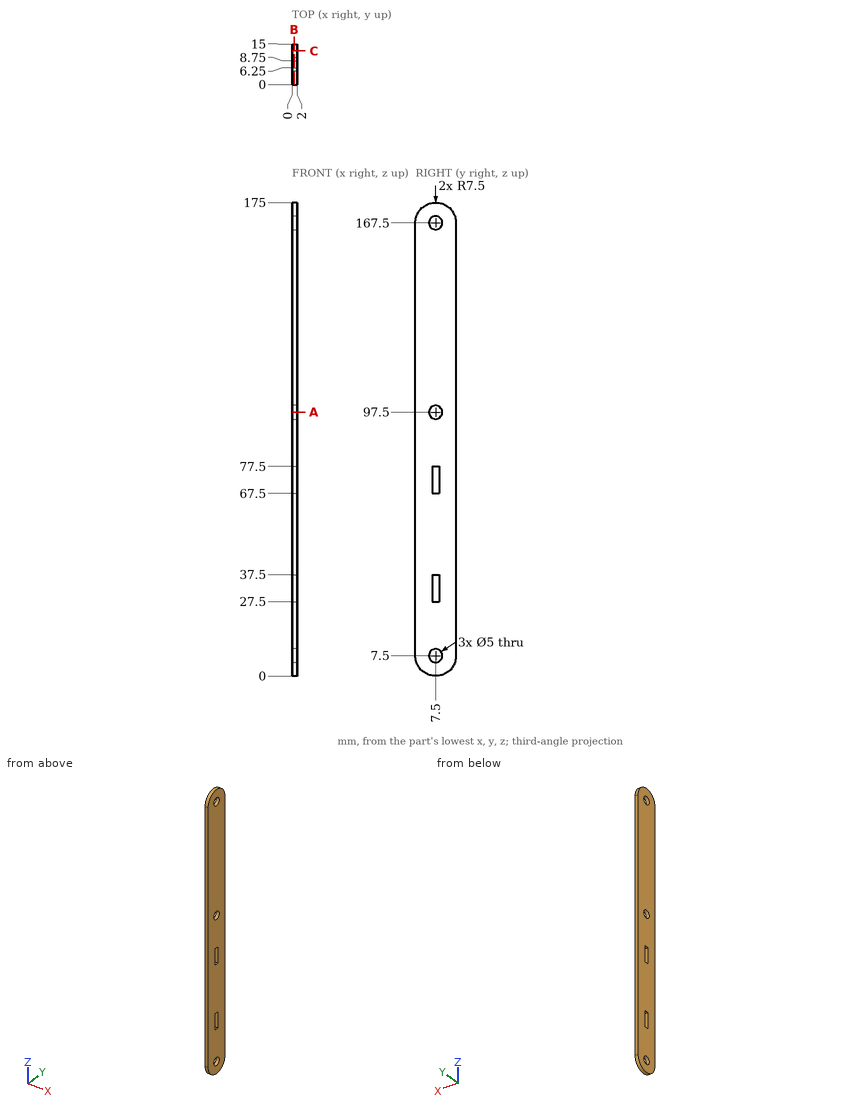
Source: three-view drawing plus pictorial views. Frame: mm from the lowest corner of the part. Give positions to 0.01 mm unless a question says otherwise; leave off trailing zeros. Write each loop counter-clockwise with the first axis right and the second up, starting at its lowest first coordinate (ties: lowest second). Pieces come first, ordered by that corner, then holes. Notation, with made-up numbers: (-10.5, 70) - (32.5, 70) arc R25 ccw to (32.5, 92) - close; hole circle Ø2 at (-34, 64). An arc over 180 degrees is marked (long way). Write item = value, one per line. Start each with the question number.
Q1. Cut plane B-B, the plane x = 0.75. Return loops of the section in (y, z), then the cut area to 3 significant figures.
Q2. Material intervals for probe 1 along Y at (x, z) = (1.1, 167.5); probe 2 along Z at (x, y) = (0.75, 6); probe 3 along Y at (x, z) = (0.15, 28), sorted ascending.
Q3. Cut plane C-C, the plane y = 12.5. Return loops of the section in (x, z), then the cut area to 3 significant figures.
Q4. Pin query (flat end, axial travel): pin 1 Ø0.6 at (x, y) = (1, 8) entering from -Z; pin 2 Ø6.5 at (y, z) = (7.5, 97.5) entering from +X. Return the tip coordinate at first contact, or that it passes through.
Q5. Cut plane A-A, the plane z = 97.5. Return loops of the section in (x, y).
Computed values:
q1.outline = (0, 7.5) arc R7.5 ccw to (15, 7.5) - (15, 167.5) arc R7.5 ccw to (0, 167.5) - close; hole circle Ø5 at (7.5, 7.5); hole circle Ø5 at (7.5, 97.5); hole circle Ø5 at (7.5, 167.5); hole (6.25, 27.5) - (8.75, 27.5) - (8.75, 37.5) - (6.25, 37.5) - close; hole (6.25, 67.5) - (8.75, 67.5) - (8.75, 77.5) - (6.25, 77.5) - close
q1.area = 2,470 mm²
q2.probe_1 = 0 to 5, 10 to 15
q2.probe_2 = 0.15 to 5.5, 9.5 to 95.5, 99.5 to 165.5, 169.5 to 174.85
q2.probe_3 = 0 to 6.25, 8.75 to 15
q3.outline = (0, 1.91) - (2, 1.91) - (2, 173.09) - (0, 173.09) - close
q3.area = 342 mm²
q4.pin_1 = 0
q4.pin_2 = 2
q5.outline = (0, 0) - (2, 0) - (2, 5) - (0, 5) - close; (0, 10) - (2, 10) - (2, 15) - (0, 15) - close
